Read the model definition and answer for the solid it produces. Units are mm, in the model's axes. A direction names the side the tool comes from. Give positions to 0.01 mm unless a question says otherwise; leave off trailing zeros. Loops run counter-clockwise (first coordinate to the right, second up) from the corner with the lowest first, then second, coordinate; pieces in that order, holes last. Notation, with made-up numbers: (88.25, 45) - (125.25, 45) arc R28 ccw to (125.25, 73) - close; hole circle Ø4 at (0, 78.5). An arc over 180 degrees is marked (long way). Write item = value, one per line. Start each with the question number.
from build123d import *

# Parameters (mm, degrees)
SKETCH_W        = 67.5
SKETCH_H        = 49
SKETCH_R        = 1.75
PAD_DEPTH       = 2
SKETCH001_W     = 67.5
SKETCH001_H     = 2
PAD001_DEPTH    = 7.5
PAD002_DEPTH    = 1.5
SKETCH003_R     = 1.6
POCKET_DEPTH    = 2.001
FILLET_R        = 1
SKETCH004_R     = 1.65
POCKET001_DEPTH = 9.501


with BuildPart() as part:
    # Sketch → Pad (new body)
    with BuildSketch(Plane.XZ):
        with Locations((0, 24.5)):
            Rectangle(SKETCH_W, SKETCH_H)
        with Locations((-28.75, 45.75)):
            Circle(SKETCH_R, mode=Mode.SUBTRACT)
        with Locations((-28.75, 14.25)):
            Circle(SKETCH_R, mode=Mode.SUBTRACT)
        with Locations((28.75, 45.75)):
            Circle(SKETCH_R, mode=Mode.SUBTRACT)
        with Locations((28.75, 14.25)):
            Circle(SKETCH_R, mode=Mode.SUBTRACT)
    extrude(amount=PAD_DEPTH)

    # Sketch001 (on Face9 of Pad) → Pad001 (join)
    with BuildSketch(Plane(origin=(0, 0, 0), x_dir=(1, 0, 0), z_dir=(0, 1, 0))):
        with Locations((0, -1)):
            Rectangle(SKETCH001_W, SKETCH001_H)
    extrude(amount=PAD001_DEPTH)

    # Sketch002 (on Face12 of Pad001) → Pad002 (join)
    with BuildSketch(Plane(origin=(33.75, 0, 0), x_dir=(0, 0, 1), z_dir=(1, 0, 0))):
        Polygon((2, 0), (2, -7.5), (49, 0), align=None)
    pad002 = extrude(amount=-PAD002_DEPTH)

    # Mirrored: Pad002 across YZ
    add(pad002.mirror(Plane.YZ))

    # Sketch003 (on Face13 of Mirrored) → Pocket (cut, through all)
    with BuildSketch(Plane(origin=(0, 0, 2), x_dir=(-1, 0, 0), z_dir=(0, 0, 1))):
        with Locations((-22.5, -3.75)):
            Circle(SKETCH003_R)
        with Locations((22.5, -3.75)):
            Circle(SKETCH003_R)
    extrude(amount=-POCKET_DEPTH, mode=Mode.SUBTRACT)

    # Fillet
    fillet_edges = [part.edges().sort_by_distance(p)[0] for p in [
        (0, 0, 2),
    ]]
    fillet(fillet_edges, radius=FILLET_R)

    # Sketch004 (on Face15 of Fillet) → Pocket001 (cut, through all)
    with BuildSketch(Plane.XZ.offset(2)):
        with Locations((-24.5, 44)):
            Circle(SKETCH004_R)
        with Locations((24.5, 44)):
            Circle(SKETCH004_R)
        with Locations((24.5, 16)):
            Circle(SKETCH004_R)
        with Locations((-24.5, 16)):
            Circle(SKETCH004_R)
    extrude(amount=-POCKET001_DEPTH, mode=Mode.SUBTRACT)


solid = part.part
1. Given P1, Ø1.5, axis at x = 8.5, y = 5, coming from the +Z side; P2, Ø3, axis at x = -28.75, z = 14.25, coming from the -Y side; P3, Ø5.5, axis at x = -24.5, z = 44, coming from the +Y side, each flat-ended and moving along its own axis, determine where each tip first touches the part or whether it passes through.
2. A cutting plane is placed at A-A on x = 28.75. Give the vertices of the cut face in (y, z).
3. For a pull along Z with two mould halves and no side action, classify faces 1 (the cylindrical face through (-24.026, 3.269, 1.014)), 2 (the flat face through (0, 4, 2)), 3 (the cylindrical face through (27.46, -0.99, 15.43)) as released by +Z, released by -Z, zero draft, split by the parting line, or undercut.
4. A tool of negligible diameter and unlimited length cuts with its end or side. For faces 4 (the flat face through (-32.25, 3, 20)), 5 (the flat face through (0, 3, 0)), from which of +Z, -Z, +X, -X, +Y, -Y can it reach the whole face along a straight path? Write none if from no direction.
5. A cutting plane is placed at B-B on y = 6.75. Give the vertices of the cut face in (x, z), and give its area (3 significant figures).
6. A cutting plane is placed at D-D on x = -13. Give the vertices of the cut face in (y, z).
7. Consider line 1 along Z through (x, y) = (-24.5, -1.4); line 2 along X through (y, z) = (1.5, 11); line 3 along X through (y, z) = (3.75, 0.95). Determine where each line is inside the solid, lowest interval first. Write a range as [from, to].
8. A cutting plane is placed at C-C on y = 3. Give the vertices of the cut face in (x, z), and give its area (3 significant figures).
Reply:
q1.P1 = 2
q1.P2 = through
q1.P3 = 0
q2.outline = (-2, 0) - (7.5, 0) - (7.5, 2) - (1, 2) arc R1 cw to (0, 3) - (0, 12.5) - (-2, 12.5) - close; (-2, 16) - (0, 16) - (0, 44) - (-2, 44) - close; (-2, 47.5) - (0, 47.5) - (0, 49) - (-2, 49) - close
q3.face_1 = zero draft
q3.face_2 = released by +Z
q3.face_3 = undercut
q4.face_4 = +Z, +Y
q4.face_5 = -Z, +X, -X, +Y, -Y
q5.outline = (-33.75, 0) - (33.75, 0) - (33.75, 6.7) - (32.25, 6.7) - (32.25, 2) - (-32.25, 2) - (-32.25, 6.7) - (-33.75, 6.7) - close
q5.area = 149 mm^2
q6.outline = (-2, 0) - (7.5, 0) - (7.5, 2) - (1, 2) arc R1 cw to (0, 3) - (0, 49) - (-2, 49) - close
q7.line_1 = [0, 14.35], [17.65, 42.35], [45.65, 49]
q7.line_2 = [-33.75, -32.25], [32.25, 33.75]
q7.line_3 = [-33.75, -24.1], [-20.9, 20.9], [24.1, 33.75]
q8.outline = (-33.75, 0) - (-23.91, 0) - (-23.91, 2) - (-32.25, 2) - (-32.25, 30.2) - (-33.75, 30.2) - close; (-21.09, 0) - (21.09, 0) - (21.09, 2) - (-21.09, 2) - close; (23.91, 0) - (33.75, 0) - (33.75, 30.2) - (32.25, 30.2) - (32.25, 2) - (23.91, 2) - close
q8.area = 208 mm^2
